The model under review builds one solid part; all positions refer to its coordinate system, in mm. A direction names the side the tool comes from. Coordinates: 2 decimals unless noted, no trailing zeros. Loops run counter-clockwise (first coordinate to the right, second up) from the corner with the lowest first, then second, coordinate; pieces in that order, holes last. Notation, with made-up numbers: M 8.25,-27.75 L 45.25,-27.75 A28 cw 45.25,3.25 Z; hole C 56,84.25 d8. An arc over 180 degrees is marked long. One line per item, written item: value.
```python
from build123d import *

# Parameters (mm, degrees)
SKIZZE1_W                       = 107
SKIZZE1_H                       = 20
AUFSATZ_LINEAR_AUSTRAGEN1_DEPTH = 12
F_7_0_7_DURCHMESSER_BOHRUNG1_D  = 7
M5_GEWINDEBOHRUNG1_D            = 4.2
M5_GEWINDEBOHRUNG2_D            = 4.2
M5_GEWINDEBOHRUNG2_DEPTH        = 10
M5_GEWINDEBOHRUNG2_TIP          = 1.2618073


with BuildPart() as part:
    # Skizze1 → Aufsatz-Linear austragen1 (new body)
    with BuildSketch(Plane.XY):
        with Locations((53.5, 10)):
            Rectangle(SKIZZE1_W, SKIZZE1_H)
    extrude(amount=AUFSATZ_LINEAR_AUSTRAGEN1_DEPTH)

    # Ø7.0 (7) Durchmesser Bohrung1 (through all)
    with Locations(Plane.XY.offset(12)):
        with Locations((17, 10), (29, 10), (41, 10)):
            Hole(F_7_0_7_DURCHMESSER_BOHRUNG1_D / 2)

    # M5 Gewindebohrung1 (through all)
    with Locations(Plane(origin=(0, 20, 0), x_dir=(1, 0, 0), z_dir=(0, 1, 0))):
        with Locations((6, -6), (101, -6), (87, -6), (57, -6)):
            Hole(M5_GEWINDEBOHRUNG1_D / 2)

    # M5 Gewindebohrung2
    with Locations(Plane(origin=(0, 20, 0), x_dir=(1, 0, 0), z_dir=(0, 1, 0))):
        with Locations((17, -6), (29, -6), (41, -6)):
            Hole(M5_GEWINDEBOHRUNG2_D / 2, depth=M5_GEWINDEBOHRUNG2_DEPTH)
            with Locations((0, 0, -(M5_GEWINDEBOHRUNG2_DEPTH + M5_GEWINDEBOHRUNG2_TIP / 2))):  # 118° drill point
                Cone(0, M5_GEWINDEBOHRUNG2_D / 2, M5_GEWINDEBOHRUNG2_TIP, mode=Mode.SUBTRACT)


solid = part.part
```
(1) Add section D-D on x = 41. State the section outline as (y, z) points.
Checks:
outline: M 0,0 L 6.5,0 L 6.5,12 L 0,12 Z; M 13.5,0 L 20,0 L 20,3.9 L 13.5,3.9 Z; M 13.5,8.1 L 20,8.1 L 20,12 L 13.5,12 Z
(2) Tool access review of faces 1 (the face through (6.46, 9.86, 8.05)), 2 (the face through (31.1, 16.35, 5.91)): name each direction out of +Z, -Z, +X, -X, +Y, -Y from which nothing blocks a thin tool from reaching the whole face with its end or side.
Checks:
face 1: +Y, -Y
face 2: +Y
(3) Add section C-C on z = 6. State how many separate pieces and enclosed holes the cut face has, then the cut area to 3 significant figures.
Checks:
separate pieces: 5
enclosed holes: 0
area: 1,600 mm^2
(4) Draft analysis for pull direction Y (two halves, no side actions). For faces 3 (the face through (107, 10, 6)), 4 (the face through (41.759, 6.583, 5.916)), 5 (the face through (53, 20, 6)), state which applies: pulls with the +Y half, pulls with the -Y half, needs draft (parallel to the pull), parting line crosses it, or undercut.
Checks:
face 3: needs draft
face 4: undercut
face 5: pulls with the +Y half
(5) Add section B-B on x = 101. State the section outline as (y, z) points, then the cut area to 3 significant figures.
Checks:
outline: M 0,0 L 20,0 L 20,3.9 L 0,3.9 Z; M 0,8.1 L 20,8.1 L 20,12 L 0,12 Z
area: 156 mm^2
(6) Insertion check: pin 1 Ø4 at (x, z) = (6, 6) entering from -Y. The pin has a flat end and moves straight along its axis. Give the tip position at first contact, or say it passes through.
Checks:
pin 1: through
(7) Add section A-A on y = 10. State the section outline as (x, z) points, then the cut area to 3 significant figures.
Checks:
outline: M 0,0 L 13.5,0 L 13.5,12 L 0,12 Z; M 20.5,0 L 25.5,0 L 25.5,12 L 20.5,12 Z; M 32.5,0 L 37.5,0 L 37.5,12 L 32.5,12 Z; M 44.5,0 L 107,0 L 107,12 L 44.5,12 Z; hole C 6,6 d4.2; hole C 57,6 d4.2; hole C 87,6 d4.2; hole C 101,6 d4.2
area: 977 mm^2
(8) To check wall thickness, follow L1, parallel to X at y = 9.75, z = 8.75; L2, parallel to Z at x = 41, y = 17; L3, parallel to X at y = 9, z = 11. State the ranges of each line that lie inside material, in increasing order. Write a range as [from, to].
Checks:
L1: [0, 13.51], [20.49, 25.51], [32.49, 37.51], [44.49, 107]
L2: [0, 3.9], [8.1, 12]
L3: [0, 13.65], [20.35, 25.65], [32.35, 37.65], [44.35, 107]
